from build123d import *

# Parameters (mm, degrees)
SKETCH_W            = 104.8
SKETCH_H            = 31
PAD_DEPTH           = 1.5
HOLE_D              = 3.4
HOLE_DEPTH          = 25
HOLE_CSINK_D        = 6.1
HOLE_CSINK_ANGLE    = 90
FILLET_R            = 3.5
SKETCH002_R         = 5.75
POCKET_DEPTH        = 1.501
LINEARPATTERN_COUNT = 2
LINEARPATTERN_PITCH = 78.74


with BuildPart() as part:
    # Sketch → Pad (new body)
    with BuildSketch(Plane.XZ):
        Rectangle(SKETCH_W, SKETCH_H)
    extrude(amount=PAD_DEPTH)

    # Hole
    with Locations(Plane.XZ.offset(1.5)):
        with Locations((-48.5, 11.5), (-48.5, -11.5), (48.5, -11.5), (48.5, 11.5)):
            CounterSinkHole(HOLE_D / 2, HOLE_CSINK_D / 2, depth=HOLE_DEPTH, counter_sink_angle=HOLE_CSINK_ANGLE)

    # Fillet
    fillet_edges = [part.edges().sort_by_distance(p)[0] for p in [
        (-52.4, -0.75, 15.5),
        (52.4, -0.75, 15.5),
    ]]
    fillet(fillet_edges, radius=FILLET_R)

    # Sketch002 (on Face5 of Fillet) → Pocket (cut, through all)
    with BuildSketch(Plane.XZ.offset(1.5)):
        with Locations((-39.37, 2.83)):
            Circle(SKETCH002_R)
    pocket = extrude(amount=-POCKET_DEPTH, mode=Mode.SUBTRACT)

    # LinearPattern: Pocket ×2
    with Locations(*[(i * LINEARPATTERN_PITCH, 0, 0) for i in range(1, LINEARPATTERN_COUNT)]):
        add(pocket, mode=Mode.SUBTRACT)


solid = part.part
Could you check a few things on this model? Use its own coordinates, in mm. Coordinates: 2 decimals unless noted, no trailing zeros. Order: outer loops, then holes, each group sorted by start corner. A loop starts at its lowest first (then second) coordinate and runs counter-clockwise, first axis right, second up. Notation, with made-up numbers: (84, 65) -> (97, 65) arc R34 ccw to (97, 102) -> close; hole circle Ø3 at (19, 65.5). An arc over 180 degrees is marked (long way). One line per item, written item: value. Start each with the question number.
1) If I drill on L1, parallel to Z at x = -48.5, y = -0.1; L2, parallel to X at y = -0.1, z = -11.5; L3, parallel to X at y = -1.15, z = 6.5, over which ranges is the centre line in solid material (lowest first)? Write a range as [from, to].
2) We'd pull the mould along X, two halves only. Please class faces 1 (the cylindrical face through (-45.114, -0.76, 3.083)), 2 (the flat face through (-1, -1.5, 0)), 3 (the cylindrical face through (51.4, -0.76, 14.45)), 4 (the cylindrical face through (44.854, -0.76, 4.557)): +X half, -X half, draft (parallel to the pull), parting line (faces both ways), or undercut.
3) I'm going to push flat-ended pins straight in: pin 1 (5.5 mm diameter, centred on x = -48.5, z = 11.5, fed in from -Y); pin 2 (10.5 mm diameter, centred on x = -39.37, z = 2.83, fed in from -Y); pin 3 (4 mm diameter, centred on x = -48.5, z = -11.5, fed in from -Y); pin 4 (2 mm diameter, centred on x = 24, z = 1.5, fed in from +Y). Where does each tip first touch, or does it pass through?
4) Imagine slicing it at B-B on x = -39.37. List the corners of the cut face in (y, z) for me.
5) Imagine slicing it at C-C on z = 2.83. List the corners of the cut face in (x, y) for me.
6) Imagine slicing it at A-A on z = -11.5. List the corners of the cut face in (x, y) for me, plus the area to 3 significant figures.
Answer list:
1. L1: z = [-15.5, -13.2], [-9.8, 9.8], [13.2, 15.5]
1. L2: x = [-52.4, -50.2], [-46.8, 46.8], [50.2, 52.4]
1. L3: x = [-52.4, -43.8], [-34.94, 34.94], [43.8, 52.4]
2. face 1: undercut
2. face 2: draft
2. face 3: +X half
2. face 4: undercut
3. pin 1: stops at y = -1.2
3. pin 2: passes through
3. pin 3: stops at y = -0.45
3. pin 4: stops at y = 0
4. outline: (-1.5, -15.5) -> (0, -15.5) -> (0, -2.92) -> (-1.5, -2.92) -> close; (-1.5, 8.58) -> (0, 8.58) -> (0, 15.5) -> (-1.5, 15.5) -> close
5. outline: (-52.4, -1.5) -> (-45.12, -1.5) -> (-45.12, 0) -> (-52.4, 0) -> close; (-33.62, -1.5) -> (33.62, -1.5) -> (33.62, 0) -> (-33.62, 0) -> close; (45.12, -1.5) -> (52.4, -1.5) -> (52.4, 0) -> (45.12, 0) -> close
6. outline: (-52.4, -1.5) -> (-51.55, -1.5) -> (-50.2, -0.15) -> (-50.2, 0) -> (-52.4, 0) -> close; (-46.8, -0.15) -> (-45.45, -1.5) -> (45.45, -1.5) -> (46.8, -0.15) -> (46.8, 0) -> (-46.8, 0) -> close; (50.2, -0.15) -> (51.55, -1.5) -> (52.4, -1.5) -> (52.4, 0) -> (50.2, 0) -> close
6. area: 143 mm2
